Design review of the part shown in the three views and the two pictorial views. Dimensions are in mm from the part's minimum x, y and z. A direction names the side the tool comes from. Coordinates: 2 decimals unless noted, no trailing zeros. Loops run counter-clockwise (first coordinate to the right, second up) from the corner with the lowest first, then second, coordinate; pieces in that order, holes last. Notation, with made-up numbers: (74, 17.5) -> (133, 17.5) arc R15 ccw to (133, 41.5) -> close; hole circle Ø6 at (-34.5, 9.5). An arc over 180 degrees is marked (long way). Use a Markdown table: item, result. Add a question column.
Q1. Take a section at A-A on z = 16. Write out the cut boundary in (x, y).
Q2. Take a section at C-C on y = 10.75. Write out the cut boundary in (x, z), plus the area to 3 significant figures.
Q3. For probe 1 along Z at (x, y) = (16, 6); probe 2 along Z at (x, y) = (12, 10.25), list the stretches that pass through material, from the lowest coordinate up.
Q4. Take a section at B-B on x = 16. Write out the cut boundary in (y, z), plus the area to 3 significant figures.
Q5. For the marked faces 4 and 5, list the 3-axis set-ups (+Z, -Z, +X, -X, +Y, -Y) from which the entire face can be reached by the end or side of a thin tool; tool diameter is ignored.
Q6. Draft analysis for pull direction X (two halves, no side actions). For the marked faces 1, 2 and 3, state which applies: pulls with the +X half, pulls with the -X half, needs draft (parallel to the pull), parting line crosses it, or undercut.
Q7. Take a section at D-D on y = 2.75. Write out the cut boundary in (x, z), plus the area to 3 significant figures.
Q8. Clearance check with flat-ended pins moving along their axes: pin 1 Ø2 at (x, y) = (8.5, 8) entering from -Z; pin 2 Ø1 at (y, z) = (6, 9) entering from -X; pin 3 Ø3 at (y, z) = (3.5, 21.5) entering from -X. State where each tip first meets the part, or that it passes through.
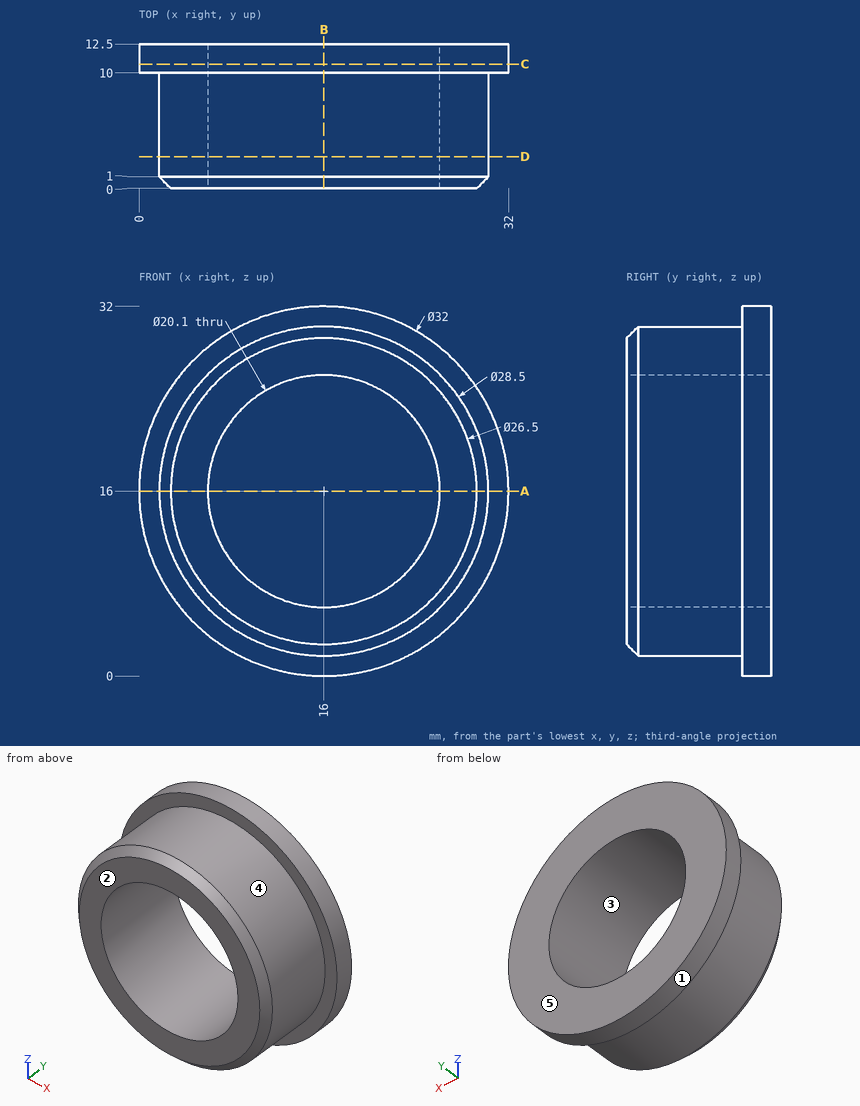
Answer list:
| question | item | result |
|---|---|---|
| 1 | outline | (0, 10) -> (1.75, 10) -> (1.75, 1) -> (2.75, 0) -> (5.95, 0) -> (5.95, 12.5) -> (0, 12.5) -> close; (26.05, 0) -> (29.25, 0) -> (30.25, 1) -> (30.25, 10) -> (32, 10) -> (32, 12.5) -> (26.05, 12.5) -> close |
| 2 | outline | circle Ø32 at (16, 16); hole circle Ø20.1 at (16, 16) |
| 2 | area | 487 mm² |
| 3 | probe 1 | 1.75 to 5.95, 26.05 to 30.25 |
| 3 | probe 2 | 0.51 to 6.78, 25.22 to 31.49 |
| 4 | outline | (0, 2.75) -> (1, 1.75) -> (10, 1.75) -> (10, 0) -> (12.5, 0) -> (12.5, 5.95) -> (0, 5.95) -> close; (0, 26.05) -> (12.5, 26.05) -> (12.5, 32) -> (10, 32) -> (10, 30.25) -> (1, 30.25) -> (0, 29.25) -> close |
| 4 | area | 113 mm² |
| 5 | face 4 | -Y |
| 5 | face 5 | +Z, -Z, +X, -X, +Y |
| 6 | face 1 | parting line crosses it |
| 6 | face 2 | needs draft |
| 6 | face 3 | undercut |
| 7 | outline | circle Ø28.5 at (16, 16); hole circle Ø20.1 at (16, 16) |
| 7 | area | 321 mm² |
| 8 | pin 1 | z = 3.32 |
| 8 | pin 2 | x = 3.32 |
| 8 | pin 3 | x = 2.32 |
